Verification items for this drawing (mm, ordinates from the low corner). A direction names the side the tool comes from. Coordinates: 2 decimals unless noted, no trailing zeros. Order: outer loops, then holes, each group sorted by start corner. A loop starts at its lowest first (then second) coordinate and runs counter-clockwise, first axis right, second up. Notation, with made-up numbers: M 67.25,-24.5 L 101.25,-24.5 A8 cw 101.25,-18.5 Z; hole C 6.25,-1.75 d10. An arc over 180 degrees is marked long. Answer as a JSON object with one key per item and string values. Group by question number.
(1) Cross-section at A-A (y = 14.5). Enter the section's corners in (x, z), plus the area to 3 significant figures.
(2) Cross-section at B-B (z = 90). Enter the section's corners in (x, y) (1 decimal).
(3) Cross-section at D-D (x = 54.5). Enter the section's corners in (y, z).
(4) Mould release check, pull along Z, two halves, no side actions. Record for the marked faces 1, 2, 3 and 4: released by +Z, released by -Z, zero draft, split by the parting line, or undercut.
(5) Cross-section at C-C (y = 50). Enter the section's corners in (x, z), plus the area to 3 significant figures.
(6) Material ranges on line 1 (Y direction, x = 4, z = 20); line 2 (Y direction, x = 11, z = 65); line 3 (X direction, y = 60, z = 75), recorded low to high.
(7) Gauge pin test, flat ends, axial feed: pin 1 Ø11 at (y, z) = (50, 20) entering from -X; pin 2 Ø4.5 at (x, z) = (97, 63.5) entering from -Y; pin 3 Ø1.5 at (y, z) = (59.5, 93.5) entering from +X; pin 4 Ø6 at (x, y) = (98, 20.5) entering from +Z. Record the tip position at first contact, or that the pin passes through.
(8) Access from +Z, -Z, +X, -X, +Y, -Y to the whole of each face (thin tool, end or side, straight path). Record for the marked faces 5, 6, 7, 8 and 9.
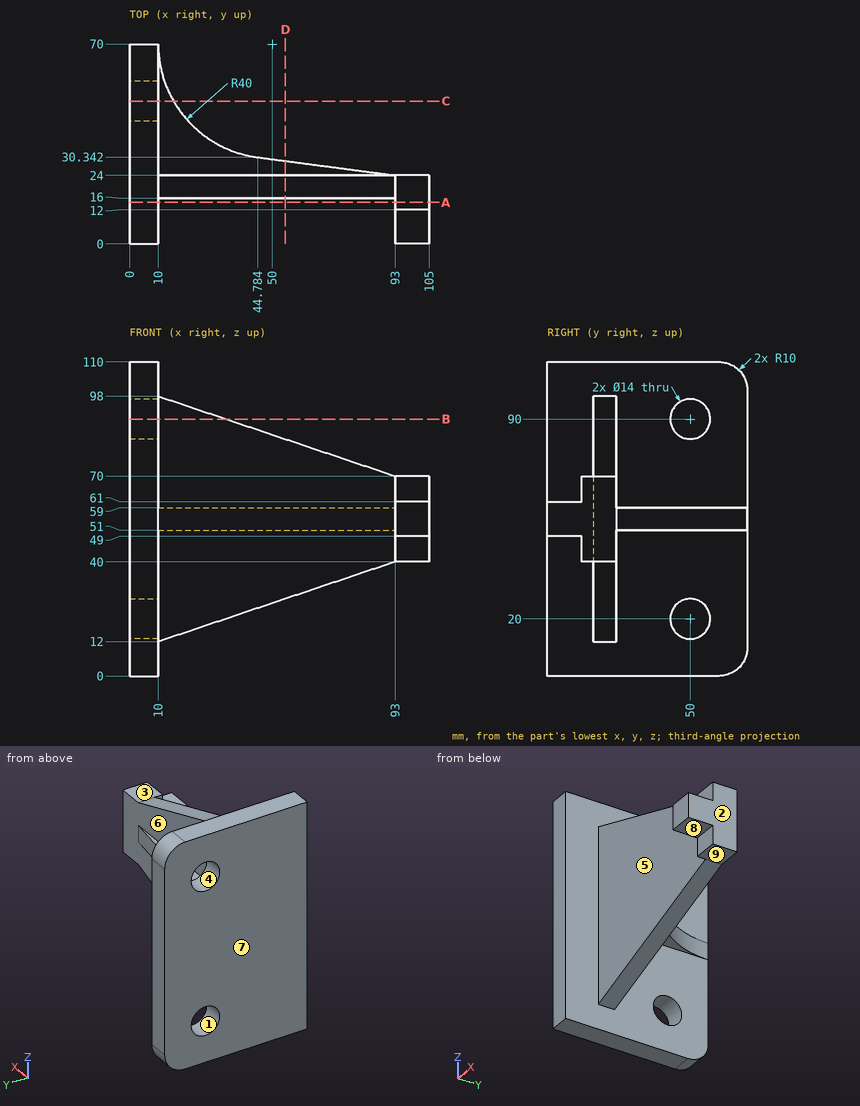
Taken from the geometry:
{
 "1": {"outline": "M 0,0 L 10,0 L 10,110 L 0,110 Z; M 93,40 L 105,40 L 105,70 L 93,70 Z", "area": "1,460 mm²"},
 "2": {"outline": "M 0,0 L 10,0 L 10,16 L 33.7,16 L 33.7,24 L 10,24 L 10,43 L 0,43 Z; M 0,57 L 10,57 L 10,70 L 0,70 Z"},
 "3": {"outline": "M 16,27.01 L 24,27.01 L 24,51 L 29.06,51 L 29.06,59 L 24,59 L 24,82.99 L 16,82.99 Z"},
 "4": {"face 1": "undercut", "face 2": "zero draft", "face 3": "released by +Z", "face 4": "undercut"},
 "5": {"outline": "M 0,0 L 10,0 L 10,13 L 0,13 Z; M 0,27 L 10,27 L 10,51 L 15.36,51 L 15.36,59 L 10,59 L 10,83 L 0,83 Z; M 0,97 L 10,97 L 10,110 L 0,110 Z", "area": "863 mm²"},
 "6": {"line 1": "y = 0 to 43, 57 to 70", "line 2": "y = 16 to 24", "line 3": "x = 0 to 10"},
 "7": {"pin 1": "passes through", "pin 2": "stops at y = 12", "pin 3": "stops at x = 10", "pin 4": "stops at z = 70"},
 "8": {"face 5": "+Z, -Z, -Y", "face 6": "+X, +Y", "face 7": "+Z, -Z, -X, +Y, -Y", "face 8": "-Z, +X, -Y", "face 9": "-Z, +X, +Y, -Y"}
}
